Check sheet for the modelled part. Datum: model origin and axes. Units: mm. Face numbers are marked on the shaded views. A direction names the side the tool comes from. Give positions to 0.01 mm unless a question says otherwise; leave off trailing zeros. Loops run counter-clockwise (first coordinate to the right, second up) from the corner with the lowest first, then second, coordinate; pieces in that order, holes last.
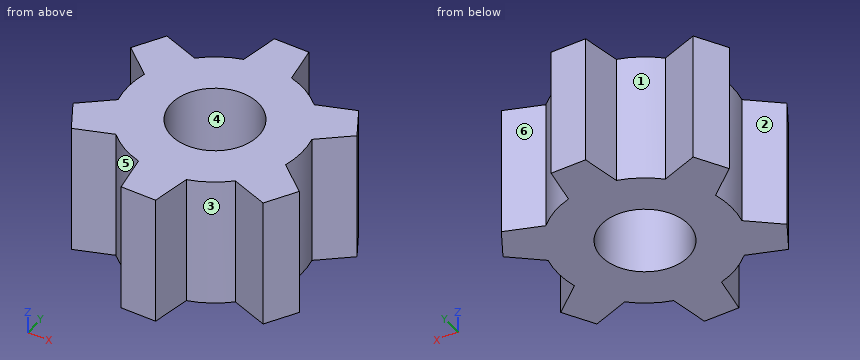
```python
from build123d import *

# Parameters (mm, degrees)
CROQUIS1_R              = 2.5
SALIENTE_EXTRUIR5_DEPTH = 7.5


with BuildPart() as part:
    # Croquis1 → Saliente-Extruir5 (new body)
    with BuildSketch(Plane.XY):
        with BuildLine():
            Line((-1, 7), (1, 7))
            Line((1, 7), (1.387053768, 4.803757055))
            ThreePointArc((1.387053768, 4.803757055), (2.5, 4.330127019), (3.466648759, 3.603102327))
            Line((3.466648759, 3.603102327), (5.562177826, 4.366025404))
            Line((5.562177826, 4.366025404), (6.562177826, 2.633974596))
            Line((6.562177826, 2.633974596), (4.853702527, 1.200654728))
            ThreePointArc((4.853702527, 1.200654728), (5, 0), (4.853702527, -1.200654728))
            Line((4.853702527, -1.200654728), (6.562177826, -2.633974596))
            Line((6.562177826, -2.633974596), (5.562177826, -4.366025404))
            Line((5.562177826, -4.366025404), (3.466648759, -3.603102327))
            ThreePointArc((3.466648759, -3.603102327), (2.5, -4.330127019), (1.387053768, -4.803757055))
            Line((1.387053768, -4.803757055), (1, -7))
            Line((1, -7), (-1, -7))
            Line((-1, -7), (-1.387053768, -4.803757055))
            ThreePointArc((-1.387053768, -4.803757055), (-2.5, -4.330127019), (-3.466648759, -3.603102327))
            Line((-3.466648759, -3.603102327), (-5.562177826, -4.366025404))
            Line((-5.562177826, -4.366025404), (-6.562177826, -2.633974596))
            Line((-6.562177826, -2.633974596), (-4.853702527, -1.200654728))
            ThreePointArc((-4.853702527, -1.200654728), (-5, 0), (-4.853702527, 1.200654728))
            Line((-4.853702527, 1.200654728), (-6.562177826, 2.633974596))
            Line((-6.562177826, 2.633974596), (-5.562177826, 4.366025404))
            Line((-5.562177826, 4.366025404), (-3.466648759, 3.603102327))
            ThreePointArc((-3.466648759, 3.603102327), (-2.5, 4.330127019), (-1.387053768, 4.803757055))
            Line((-1.387053768, 4.803757055), (-1, 7))
        make_face()
        Circle(CROQUIS1_R, mode=Mode.SUBTRACT)
    extrude(amount=SALIENTE_EXTRUIR5_DEPTH)


solid = part.part
```
(1) Section check B-B on x = 0. Record the boundary of the cut face in (y, z), plus the area to 3 significant figures.
(2) Gauge pin test, flat ends, axial feed: pin 1 Ø3 at (y, z) = (-1, 2.5) entering from +X; pin 2 Ø2 at (y, z) = (5, 5) entering from -X. Record the tip position at first contact, or that the pin passes through.
(3) Material ranges on line 1 (Y direction, x = 0, z = 4.75); line 2 (Y direction, x = 2.25, z = 2); line 3 (X direction, y = 1.25, z = 6.25), recorded low to high.
(4) Section check D-D on y = 6. Record the boundary of the cut face in (x, z).
(5) Section check A-A on y = 0. Record the boundary of the cut face in (x, z).
(6) Access from +Z, -Z, +X, -X, +Y, -Y to the whole of each face (thin tool, end or side, straight path). Record for the marked faces 1, 2 and 3.
(7) Release check for a two-part mould opening along Y. For the marked faces 4, 5 and 6 record: pulls with the +Y half, pulls with the -Y half, needs draft (parallel to the pull), parting line crosses it, or undercut.
(8) Section check C-C on z = 1.25. Record the boundary of the cut face in (x, y), plus the area to 3 significant figures.
Computed values:
1. outline: (-7, 0) - (-2.5, 0) - (-2.5, 7.5) - (-7, 7.5) - close; (2.5, 0) - (7, 0) - (7, 7.5) - (2.5, 7.5) - close
1. area: 67.5 mm2
2. pin 1: stops at x = 6.4
2. pin 2: stops at x = -5.77
3. line 1: y = -7 to -2.5, 2.5 to 7
3. line 2: y = -4.47 to -1.09, 1.09 to 4.47
3. line 3: x = -4.91 to -2.17, 2.17 to 4.91
4. outline: (-1.18, 0) - (1.18, 0) - (1.18, 7.5) - (-1.18, 7.5) - close
5. outline: (-5, 0) - (-2.5, 0) - (-2.5, 7.5) - (-5, 7.5) - close; (2.5, 0) - (5, 0) - (5, 7.5) - (2.5, 7.5) - close
6. face 1: +Z, -Z, +Y
6. face 2: +Z, -Z, -X
6. face 3: +Z, -Z, -Y
7. face 4: undercut
7. face 5: pulls with the -Y half
7. face 6: pulls with the +Y half
8. outline: (-6.56, -2.63) - (-5.56, -4.37) - (-3.47, -3.6) arc R5 ccw to (-1.39, -4.8) - (-1, -7) - (1, -7) - (1.39, -4.8) arc R5 ccw to (3.47, -3.6) - (5.56, -4.37) - (6.56, -2.63) - (4.85, -1.2) arc R5 ccw to (4.85, 1.2) - (6.56, 2.63) - (5.56, 4.37) - (3.47, 3.6) arc R5 ccw to (1.39, 4.8) - (1, 7) - (-1, 7) - (-1.39, 4.8) arc R5 ccw to (-3.47, 3.6) - (-5.56, 4.37) - (-6.56, 2.63) - (-4.85, 1.2) arc R5 ccw to (-4.85, -1.2) - close; hole circle Ø5 at (0, 0)
8. area: 88.2 mm2
